Input: part model. Units: mm. Frame: model coordinates. A direction names the side the tool comes from. Coordinates: 2 decimals unless noted, no trailing zeros. Write each loop counter-clockwise with the first axis right and the second up, starting at its lowest first coordinate (ties: lowest second). Pieces come first, ordered by that corner, then holes. Notation, with made-up numbers: (48.5, 88) - (76.5, 88) arc R28 ccw to (76.5, 116) - close; hole circle Ø10 at (-20, 28.25). An arc over 180 degrees is marked (long way). Use a Markdown table: item, result. Add a question column.
Q1. Section query A-A (x = -1.25). Return the cut outline in (y, z).
Q2. Pin query (flat end, axial travel): P1, Ø1, axis at x = -2, z = 77.5, coming from the -Y side; P2, Ø5, axis at y = 0, z = 57, coming from the -X side; P3, Ø0.8, axis at x = 9, z = 24, coming from the +Y side. Return the tip coordinate at first contact, or that it passes through.
Q3. Set-up query: faces 1 (the face through (-4.023, 0, 44)), 2 (the face through (-8.323, -4, 44)), 3 (the face through (3.777, 0, 44)). Return all of +Z, -Z, +X, -X, +Y, -Y with unobstructed straight access to the full face (end or side cutting, diameter ignored); none if empty.
Q4. Material intervals for probe 1 along X at (y, z) = (0, 76); probe 2 along Y at (x, z) = (4.5, 43.5); probe 3 along X at (y, z) = (-3.5, 39.5), sorted ascending. Write a range as from..to.
Q5. Mould query, pull axis Y, two halves, no side actions, for faces 4 (the face through (2, 2, 90)), 5 (the face through (-6, 9.965, 44)), 6 (the face through (4, -8.235, 44)). Classes: released by +Y, released by -Y, zero draft, split by the parting line, or undercut.
from build123d import *

# Parameters (mm, degrees)
SKETCH_1_R      = 2.5
EXTRUDE_1_DEPTH = 90


with BuildPart() as part:
    # 草图1 → 凸台-拉伸1 (new body)
    with BuildSketch(Plane.XY):
        with BuildLine():
            Line((4.215995631, 3.244230202), (6.436655803, 5.464890373))
            Line((6.436655803, 5.464890373), (7.776655803, 5.464890373))
            ThreePointArc((7.776655803, 5.464890373), (7.988787838, 5.377022408), (8.076655803, 5.164890373))
            Line((8.076655803, 5.164890373), (8.076655803, 3.364890373))
            ThreePointArc((8.076655803, 3.364890373), (8.164523769, 3.152758339), (8.376655803, 3.064890373))
            Line((8.376655803, 3.064890373), (9.376655803, 3.064890373))
            Line((9.376655803, 3.064890373), (9.376655803, 3.364890373))
            ThreePointArc((9.376655803, 3.364890373), (9.435234447, 3.50631173), (9.576655803, 3.564890373))
            Line((9.576655803, 3.564890373), (9.876655803, 3.564890373))
            Line((9.876655803, 3.564890373), (9.876655803, 8.464890373))
            ThreePointArc((9.876655803, 8.464890373), (9.437315975, 9.525550545), (8.376655803, 9.964890373))
            Line((8.376655803, 9.964890373), (3.476655803, 9.964890373))
            Line((3.476655803, 9.964890373), (3.476655803, 9.664890373))
            ThreePointArc((3.476655803, 9.664890373), (3.418077159, 9.523469017), (3.276655803, 9.464890373))
            Line((3.276655803, 9.464890373), (2.976655803, 9.464890373))
            Line((2.976655803, 9.464890373), (2.976655803, 8.464890373))
            ThreePointArc((2.976655803, 8.464890373), (3.064523769, 8.252758339), (3.276655803, 8.164890373))
            Line((3.276655803, 8.164890373), (5.076655803, 8.164890373))
            ThreePointArc((5.076655803, 8.164890373), (5.288787838, 8.077022408), (5.376655803, 7.864890373))
            Line((5.376655803, 7.864890373), (5.376655803, 6.524890373))
            Line((5.376655803, 6.524890373), (3.155995631, 4.304230202))
            ThreePointArc((3.155995631, 4.304230202), (2.669360608, 3.979071075), (2.09533546, 3.864890373))
            Line((2.09533546, 3.864890373), (-2.342023853, 3.864890373))
            ThreePointArc((-2.342023853, 3.864890373), (-2.916049002, 3.979071075), (-3.402684025, 4.304230202))
            Line((-3.402684025, 4.304230202), (-5.623344197, 6.524890373))
            Line((-5.623344197, 6.524890373), (-5.623344197, 7.864890373))
            ThreePointArc((-5.623344197, 7.864890373), (-5.535476231, 8.077022408), (-5.323344197, 8.164890373))
            Line((-5.323344197, 8.164890373), (-3.523344197, 8.164890373))
            ThreePointArc((-3.523344197, 8.164890373), (-3.311212162, 8.252758339), (-3.223344197, 8.464890373))
            Line((-3.223344197, 8.464890373), (-3.223344197, 9.464890373))
            Line((-3.223344197, 9.464890373), (-3.523344197, 9.464890373))
            ThreePointArc((-3.523344197, 9.464890373), (-3.664765553, 9.523469017), (-3.723344197, 9.664890373))
            Line((-3.723344197, 9.664890373), (-3.723344197, 9.964890373))
            Line((-3.723344197, 9.964890373), (-8.623344197, 9.964890373))
            ThreePointArc((-8.623344197, 9.964890373), (-9.684004369, 9.525550545), (-10.123344197, 8.464890373))
            Line((-10.123344197, 8.464890373), (-10.123344197, 3.564890373))
            Line((-10.123344197, 3.564890373), (-9.823344197, 3.564890373))
            ThreePointArc((-9.823344197, 3.564890373), (-9.681922841, 3.50631173), (-9.623344197, 3.364890373))
            Line((-9.623344197, 3.364890373), (-9.623344197, 3.064890373))
            Line((-9.623344197, 3.064890373), (-8.623344197, 3.064890373))
            ThreePointArc((-8.623344197, 3.064890373), (-8.411212162, 3.152758339), (-8.323344197, 3.364890373))
            Line((-8.323344197, 3.364890373), (-8.323344197, 5.164890373))
            ThreePointArc((-8.323344197, 5.164890373), (-8.235476231, 5.377022408), (-8.023344197, 5.464890373))
            Line((-8.023344197, 5.464890373), (-6.683344197, 5.464890373))
            Line((-6.683344197, 5.464890373), (-4.462684025, 3.244230202))
            ThreePointArc((-4.462684025, 3.244230202), (-4.137524898, 2.757595178), (-4.023344197, 2.18357003))
            Line((-4.023344197, 2.18357003), (-4.023344197, -2.253789283))
            ThreePointArc((-4.023344197, -2.253789283), (-4.137524898, -2.827814432), (-4.462684025, -3.314449455))
            Line((-4.462684025, -3.314449455), (-6.683344197, -5.535109627))
            Line((-6.683344197, -5.535109627), (-8.023344197, -5.535109627))
            ThreePointArc((-8.023344197, -5.535109627), (-8.235476231, -5.447241661), (-8.323344197, -5.235109627))
            Line((-8.323344197, -5.235109627), (-8.323344197, -3.435109627))
            ThreePointArc((-8.323344197, -3.435109627), (-8.411212162, -3.222977592), (-8.623344197, -3.135109627))
            Line((-8.623344197, -3.135109627), (-9.623344197, -3.135109627))
            Line((-9.623344197, -3.135109627), (-9.623344197, -3.435109627))
            ThreePointArc((-9.623344197, -3.435109627), (-9.681922841, -3.576530983), (-9.823344197, -3.635109627))
            Line((-9.823344197, -3.635109627), (-10.123344197, -3.635109627))
            Line((-10.123344197, -3.635109627), (-10.123344197, -8.535109627))
            ThreePointArc((-10.123344197, -8.535109627), (-9.684004369, -9.595769798), (-8.623344197, -10.035109627))
            Line((-8.623344197, -10.035109627), (-3.723344197, -10.035109627))
            Line((-3.723344197, -10.035109627), (-3.723344197, -9.735109627))
            ThreePointArc((-3.723344197, -9.735109627), (-3.664765553, -9.59368827), (-3.523344197, -9.535109627))
            Line((-3.523344197, -9.535109627), (-3.223344197, -9.535109627))
            Line((-3.223344197, -9.535109627), (-3.223344197, -8.535109627))
            ThreePointArc((-3.223344197, -8.535109627), (-3.311212162, -8.322977592), (-3.523344197, -8.235109627))
            Line((-3.523344197, -8.235109627), (-5.323344197, -8.235109627))
            ThreePointArc((-5.323344197, -8.235109627), (-5.535476231, -8.147241661), (-5.623344197, -7.935109627))
            Line((-5.623344197, -7.935109627), (-5.623344197, -6.595109627))
            Line((-5.623344197, -6.595109627), (-3.402684025, -4.374449455))
            ThreePointArc((-3.402684025, -4.374449455), (-2.916049002, -4.049290328), (-2.342023853, -3.935109627))
            Line((-2.342023853, -3.935109627), (2.09533546, -3.935109627))
            ThreePointArc((2.09533546, -3.935109627), (2.669360608, -4.049290328), (3.155995631, -4.374449455))
            Line((3.155995631, -4.374449455), (5.376655803, -6.595109627))
            Line((5.376655803, -6.595109627), (5.376655803, -7.935109627))
            ThreePointArc((5.376655803, -7.935109627), (5.288787838, -8.147241661), (5.076655803, -8.235109627))
            Line((5.076655803, -8.235109627), (3.276655803, -8.235109627))
            ThreePointArc((3.276655803, -8.235109627), (3.064523769, -8.322977592), (2.976655803, -8.535109627))
            Line((2.976655803, -8.535109627), (2.976655803, -9.535109627))
            Line((2.976655803, -9.535109627), (3.276655803, -9.535109627))
            ThreePointArc((3.276655803, -9.535109627), (3.418077159, -9.59368827), (3.476655803, -9.735109627))
            Line((3.476655803, -9.735109627), (3.476655803, -10.035109627))
            Line((3.476655803, -10.035109627), (8.376655803, -10.035109627))
            ThreePointArc((8.376655803, -10.035109627), (9.437315975, -9.595769798), (9.876655803, -8.535109627))
            Line((9.876655803, -8.535109627), (9.876655803, -3.635109627))
            Line((9.876655803, -3.635109627), (9.576655803, -3.635109627))
            ThreePointArc((9.576655803, -3.635109627), (9.435234447, -3.576530983), (9.376655803, -3.435109627))
            Line((9.376655803, -3.435109627), (9.376655803, -3.135109627))
            Line((9.376655803, -3.135109627), (8.376655803, -3.135109627))
            ThreePointArc((8.376655803, -3.135109627), (8.164523769, -3.222977592), (8.076655803, -3.435109627))
            Line((8.076655803, -3.435109627), (8.076655803, -5.235109627))
            ThreePointArc((8.076655803, -5.235109627), (7.988787838, -5.447241661), (7.776655803, -5.535109627))
            Line((7.776655803, -5.535109627), (6.436655803, -5.535109627))
            Line((6.436655803, -5.535109627), (4.215995631, -3.314449455))
            ThreePointArc((4.215995631, -3.314449455), (3.890836504, -2.827814432), (3.776655803, -2.253789283))
            Line((3.776655803, -2.253789283), (3.776655803, 2.18357003))
            ThreePointArc((3.776655803, 2.18357003), (3.890836504, 2.757595178), (4.215995631, 3.244230202))
        make_face()
        with Locations(Location((-0.123344197, -0.035109627, 0), (0, 0, 180))):
            Circle(SKETCH_1_R, mode=Mode.SUBTRACT)
    extrude(amount=EXTRUDE_1_DEPTH)


solid = part.part
Values follow:
| question | item | result |
|---|---|---|
| 1 | outline | (-3.94, 0) - (-2.27, 0) - (-2.27, 90) - (-3.94, 90) - close; (2.2, 0) - (3.86, 0) - (3.86, 90) - (2.2, 90) - close |
| 2 | P1 | y = -3.94 |
| 2 | P2 | x = -4.06 |
| 2 | P3 | y = 9.95 |
| 3 | face 1 | +Z, -Z, -X |
| 3 | face 2 | +Z, -Z |
| 3 | face 3 | +Z, -Z, +X |
| 4 | probe 1 | -4.02..-2.62, 2.38..3.78 |
| 4 | probe 2 | -10.04..-8.24, -5.72..-3.6, 3.53..5.65, 8.16..9.96 |
| 4 | probe 3 | -9.63..-8.32, -4.65..4.4, 8.08..9.39 |
| 5 | face 4 | zero draft |
| 5 | face 5 | released by +Y |
| 5 | face 6 | undercut |
